from build123d import *

# Parameters (mm, degrees)
F1_DEPTH = 4.064
F3_D     = 5.08
F4_W     = 347.472
F4_H     = 195.072
F5_DEPTH = 25.4
F7_D     = 5.08


with BuildPart() as f1:
    # F0 (on Top) → F1 (new body)
    with BuildSketch(Plane.XY):
        Polygon((181.124512, 101.6), (-174.475488, 101.6), (-174.475488, 88.9), (-174.475488, -101.6), (181.124512, -101.6), (181.124512, 88.9), align=None)
    extrude(amount=F1_DEPTH)

    # F3 (through all)
    with Locations(Plane(origin=(0, 0, 0), x_dir=(1, 0, 0), z_dir=(0, 0, -1))):
        with Locations((-166.220488, -91.44), (170.964512, -91.44), (-164.315488, 91.44), (170.964512, 91.44)):
            Hole(F3_D / 2)

    # F4 (on face) → F5 (join)
    with BuildSketch(Plane.XY.offset(4.064)):
        Polygon((181.124512, 101.6), (177.060512, 101.6), (-174.475488, 101.6), (-174.475488, -101.6), (181.124512, -101.6), align=None)
        with Locations((3.324512, 0)):
            Rectangle(F4_W, F4_H, mode=Mode.SUBTRACT)
    extrude(amount=F5_DEPTH)

    # F7 (through all)
    with Locations(Plane.XY.offset(4.064)):
        with Locations((-156.060488, -91.44), (164.614512, -91.44), (164.614512, 91.44), (-159.870488, 91.44)):
            Hole(F7_D / 2)


solid = f1.part
Check sheet for the modelled part. Datum: model origin and axes. Units: mm. A direction names the side the tool comes from. Give positions to 0.01 mm unless a question says otherwise; leave off trailing zeros. Write each loop counter-clockwise with the first axis right and the second up, starting at its lowest first coordinate (ties: lowest second). Pieces come first, ordered by that corner, then holes. Notation, with made-up numbers: (67.25, 5.5) -> (124.25, 5.5) arc R12 cw to (124.25, 23.5) -> close; hole circle Ø6 at (60.25, 63). An arc over 180 degrees is marked (long way). Use one line per item in the form item = value. Start each with the question number.
1. Access from +Z, -Z, +X, -X, +Y, -Y to the whole of each face (thin tool, end or side, straight path). Record for faces 1 (the flat face through (-170.411, -1, 17)), 2 (the flat face through (1, -101.6, 15)).
2. Mould release check, pull along X, two halves, no side actions. Record for faces 3 (the flat face through (1, 97.536, 17)), 4 (the flat face through (-174.475, 1, 15)), 5 (the flat face through (2, 98, 29.464)): pulls with the +X half, pulls with the -X half, needs draft (parallel to the pull), parting line crosses it, or undercut.
3. Section check B-B (y = 36.5). Record the cut outline in (x, z).
4. Thickness scan on line 1 along Y through (x, z) = (130, 22.5); line 2 along X through (y, z) = (-33, 5.5); line 3 along Z through (x, y) = (-110.5, 57.5). Record the ranges inside material, lowest first. Write a range as from..to.
5. Go/stop test with a flat-tipped pin: P1, Ø8, axis at x = -115.5, y = -39.5, coming from the +Z side. Record where the tip stops, or that it passes through.
6. Section check A-A (x = -108). Record the cut outline in (y, z), and give its area (3 significant figures).
Conclusion:
q1.face_1 = +Z
q1.face_2 = +Z, -Z, +X, -X, -Y
q2.face_3 = undercut
q2.face_4 = pulls with the -X half
q2.face_5 = needs draft
q3.outline = (-174.48, 0) -> (181.12, 0) -> (181.12, 29.46) -> (177.06, 29.46) -> (177.06, 4.06) -> (-170.41, 4.06) -> (-170.41, 29.46) -> (-174.48, 29.46) -> close
q4.line_1 = -101.6..-97.54, 97.54..101.6
q4.line_2 = -174.48..-170.41, 177.06..181.12
q4.line_3 = 0..4.06
q5.P1 = 4.06
q6.outline = (-101.6, 0) -> (101.6, 0) -> (101.6, 29.46) -> (97.54, 29.46) -> (97.54, 4.06) -> (-97.54, 4.06) -> (-97.54, 29.46) -> (-101.6, 29.46) -> close
q6.area = 1,030 mm²
